from build123d import *

# Parameters (mm, degrees)
BOSS_EXTRUDE1_DEPTH = 1.65
SKETCH2_R           = 1.4
CUT_EXTRUDE1_DEPTH  = 1.65


with BuildPart() as part:
    # Sketch1 → Boss-Extrude1 (new body)
    with BuildSketch(Plane.XY):
        with BuildLine():
            Line((27, -30), (-27, -30))
            ThreePointArc((-27, -30), (-29.121320344, -29.121320344), (-30, -27))
            Line((-30, -27), (-30, 27))
            ThreePointArc((-30, 27), (-29.121320344, 29.121320344), (-27, 30))
            Line((-27, 30), (27, 30))
            ThreePointArc((27, 30), (29.121320344, 29.121320344), (30, 27))
            Line((30, 27), (30, -27))
            ThreePointArc((30, -27), (29.121320344, -29.121320344), (27, -30))
        make_face()
    extrude(amount=BOSS_EXTRUDE1_DEPTH)

    # Sketch2 → Cut-Extrude1 (cut)
    with BuildSketch(Plane.XY.offset(1.65)):
        with Locations((-11.75, 26.45)):
            Circle(SKETCH2_R)
        with Locations(Location((11.75, 26.45, 0), (0, 0, 180))):
            Circle(SKETCH2_R)
        with Locations((11.75, -26.45)):
            Circle(SKETCH2_R)
        with Locations(Location((-11.75, -26.45, 0), (0, 0, 180))):
            Circle(SKETCH2_R)
        with BuildLine():
            Line((23.551533864, -23.55), (23.551533864, 23.55))
            ThreePointArc((23.551533864, 23.55), (24.6, 24.598466136), (25.648466136, 23.55))
            Line((25.648466136, 23.55), (25.648466136, -23.55))
            ThreePointArc((25.648466136, -23.55), (24.6, -24.598466136), (23.551533864, -23.55))
        make_face()
        with BuildLine():
            Line((-1.048466136, -23.55), (-1.048466136, 23.55))
            ThreePointArc((-1.048466136, 23.55), (0, 24.598466136), (1.048466136, 23.55))
            Line((1.048466136, 23.55), (1.048466136, -23.55))
            ThreePointArc((1.048466136, -23.55), (0, -24.598466136), (-1.048466136, -23.55))
        make_face()
        with BuildLine():
            Line((-25.648466136, -23.55), (-25.648466136, 23.55))
            ThreePointArc((-25.648466136, 23.55), (-24.6, 24.598466136), (-23.551533864, 23.55))
            Line((-23.551533864, 23.55), (-23.551533864, -23.55))
            ThreePointArc((-23.551533864, -23.55), (-24.6, -24.598466136), (-25.648466136, -23.55))
        make_face()
        with BuildLine():
            Line((-9.13875967, -18.55), (-9.13875967, 18.55))
            ThreePointArc((-9.13875967, 18.55), (-8.3, 19.38875967), (-7.46124033, 18.55))
            Line((-7.46124033, 18.55), (-7.46124033, -18.55))
            ThreePointArc((-7.46124033, -18.55), (-8.3, -19.38875967), (-9.13875967, -18.55))
        make_face()
        with BuildLine():
            Line((15.15, -17.55), (15.15, 17.55))
            ThreePointArc((15.15, 17.55), (17.1, 19.5), (19.05, 17.55))
            Line((19.05, 17.55), (19.05, -17.55))
            ThreePointArc((19.05, -17.55), (17.1, -19.5), (15.15, -17.55))
        make_face()
        with BuildLine():
            Line((-19.05, -17.55), (-19.05, 17.55))
            ThreePointArc((-19.05, 17.55), (-17.1, 19.5), (-15.15, 17.55))
            Line((-15.15, 17.55), (-15.15, -17.55))
            ThreePointArc((-15.15, -17.55), (-17.1, -19.5), (-19.05, -17.55))
        make_face()
        with BuildLine():
            Line((7.46124033, -18.55), (7.46124033, 18.55))
            ThreePointArc((7.46124033, 18.55), (8.3, 19.38875967), (9.13875967, 18.55))
            Line((9.13875967, 18.55), (9.13875967, -18.55))
            ThreePointArc((9.13875967, -18.55), (8.3, -19.38875967), (7.46124033, -18.55))
        make_face()
    extrude(amount=-CUT_EXTRUDE1_DEPTH, mode=Mode.SUBTRACT)


solid = part.part
Read the model definition and answer for the solid it produces. Units are mm, in the model's axes. A direction names the side the tool comes from. Round coordinates to 2 decimals unless told otherwise and drop trailing zeros. Write each loop counter-clockwise with the first axis right and the second up, starting at its lowest first coordinate (ties: lowest second). Pieces come first, ordered by that corner, then holes. Notation, with made-up numbers: (56, 44.5) - (103, 44.5) arc R37 ccw to (103, 81.5) - close; hole circle Ø1 at (-0.5, 86.5). An arc over 180 degrees is marked (long way). One line per question, with ' | ' between items. Start each with the question number.
1. This flat-tipped pin is pushed along its axis until it touches: pin 1 (2 mm diameter, centred on x = -11.75, y = -26.45, fed in from -Z). Where does it stop, or does it pass through?
2. Section B-B (y = 8) is taken. Give the number of separate pieces and of enclosed holes in the cut face, and give its area (3 significant figures).
3. Section C-C (x = -12) is taken. Determine the outline of the cut face in (y, z), and give its area (3 significant figures).
4. Section D-D (x = 24.6) is taken. Determine the outline of the cut face in (y, z).
5. Find the intervals of material crossed by probe 1 along Y at (x, z) = (11.75, 0.65); probe 2 along X at (y, z) = (21.5, 0.9); probe 3 along X at (y, z) = (-26.5, 1.2), in increasing order. Write a range as [from, to].
6. Section A-A (x = 17.1) is taken. Determine the outline of the cut face in (y, z).
7. For a pull along Y with two mould halves and no side action, classify faces 1 (the face through (7, 0, 1.65)), 2 (the face through (-8.28, -19.39, 0.84)), 3 (the face through (-29.14, 29.1, 0.81)), 4 (the face through (9.139, 0, 1)) as +Y half, -Y half, draft (parallel to the pull), parting line (faces both ways), or undercut.
8. For faces 5 (the face through (30, 0, 1)), 6 (the face through (19.05, 0, 1)), determine the directions among +Z, -Z, +X, -X, +Y, -Y from which every point of the face is accessible in a straight line to the end or side of a thin tool.
Filled in:
1) pin 1: through
2) separate pieces: 8 | enclosed holes: 0 | area: 70.2 mm²
3) outline: (-30, 0) - (-27.83, 0) - (-27.83, 1.65) - (-30, 1.65) - close; (-25.07, 0) - (25.07, 0) - (25.07, 1.65) - (-25.07, 1.65) - close; (27.83, 0) - (30, 0) - (30, 1.65) - (27.83, 1.65) - close | area: 89.9 mm²
4) outline: (-30, 0) - (-24.6, 0) - (-24.6, 1.65) - (-30, 1.65) - close; (24.6, 0) - (30, 0) - (30, 1.65) - (24.6, 1.65) - close
5) probe 1: [-30, -27.85], [-25.05, 25.05], [27.85, 30] | probe 2: [-30, -25.65], [-23.55, -1.05], [1.05, 23.55], [25.65, 30] | probe 3: [-30, -13.15], [-10.35, 10.35], [13.15, 30]
6) outline: (-30, 0) - (-19.5, 0) - (-19.5, 1.65) - (-30, 1.65) - close; (19.5, 0) - (30, 0) - (30, 1.65) - (19.5, 1.65) - close
7) face 1: draft | face 2: undercut | face 3: +Y half | face 4: undercut
8) face 5: +Z, -Z, +X, +Y, -Y | face 6: +Z, -Z
